from build123d import *

# Parameters (mm, degrees)
SKETCH1_R           = 1.75
SKETCH1_W           = 10
SKETCH1_H           = 5
SKETCH1_W_2         = 15
BOSS_EXTRUDE1_DEPTH = 5
SKETCH3_R           = 3.175
CUT_EXTRUDE1_DEPTH  = 2


with BuildPart() as part:
    # Sketch1 → Boss-Extrude1 (new body)
    with BuildSketch(Plane(origin=(0, 0, 0), x_dir=(1, 0, 0), z_dir=(0, 1, 0))):
        Polygon((3.647196653, 31.359118607), (3.647196653, 36.359118607), (13.647196653, 36.359118607), (13.647196653, 31.359118607), (53.647196653, 31.359118607), (53.647196653, 36.359118607), (63.647196653, 36.359118607), (63.647196653, 31.359118607), (93.647196653, 31.359118607), (93.647196653, 3.859118607), (63.647196653, 3.859118607), (63.647196653, -3.640881393), (93.647196653, -3.640881393), (93.647196653, -31.140881393), (63.647196653, -31.140881393), (63.647196653, -36.140881393), (53.647196653, -36.140881393), (53.647196653, -31.140881393), (13.647196653, -31.140881393), (13.647196653, -36.140881393), (3.647196653, -36.140881393), (3.647196653, -31.140881393), (-41.852803347, -31.140881393), (-41.852803347, 31.359118607), align=None)
        with Locations(Location((73.647196653, 22.609118607, 0), (0, 0, 270))):
            Circle(SKETCH1_R, mode=Mode.SUBTRACT)
        with Locations(Location((-1.352803347, 22.609118607, 0), (0, 0, 270))):
            Circle(SKETCH1_R, mode=Mode.SUBTRACT)
        with Locations(Location((73.647196653, -22.390881393, 0), (0, 0, 270))):
            Circle(SKETCH1_R, mode=Mode.SUBTRACT)
        with Locations(Location((-1.352803347, -22.390881393, 0), (0, 0, 270))):
            Circle(SKETCH1_R, mode=Mode.SUBTRACT)
        with Locations((83.647196653, -20.390881393)):
            Rectangle(SKETCH1_W, SKETCH1_H, mode=Mode.SUBTRACT)
        with Locations((-31.352803347, -22.390881393)):
            Rectangle(SKETCH1_W_2, SKETCH1_H, mode=Mode.SUBTRACT)
        with Locations((-31.352803347, 22.609118607)):
            Rectangle(SKETCH1_W_2, SKETCH1_H, mode=Mode.SUBTRACT)
        with Locations((83.647196653, 20.609118607)):
            Rectangle(SKETCH1_W, SKETCH1_H, mode=Mode.SUBTRACT)
    extrude(amount=BOSS_EXTRUDE1_DEPTH)

    # Sketch3 → Cut-Extrude1 (cut)
    with BuildSketch(Plane.XZ):
        with Locations(Location((-1.352803347, 22.390881393, 0), (0, 0, 270))):
            Circle(SKETCH3_R)
        with Locations(Location((73.647196653, 22.390881393, 0), (0, 0, 270))):
            Circle(SKETCH3_R)
        with Locations(Location((-1.352803347, -22.609118607, 0), (0, 0, 270))):
            Circle(SKETCH3_R)
        with Locations(Location((73.647196653, -22.609118607, 0), (0, 0, 270))):
            Circle(SKETCH3_R)
    extrude(amount=-CUT_EXTRUDE1_DEPTH, mode=Mode.SUBTRACT)


solid = part.part
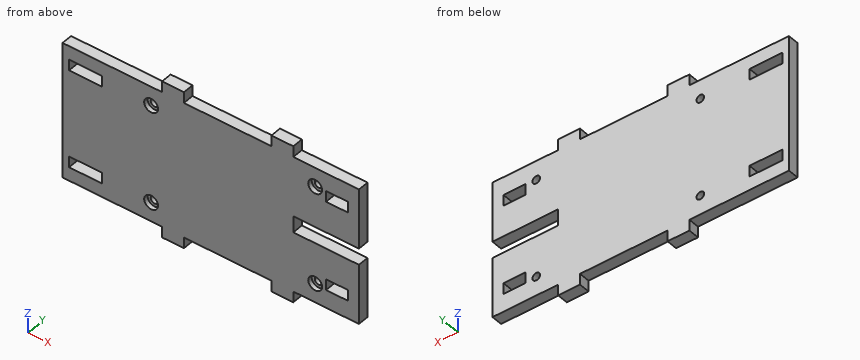
Geometry check sheet. Reference: the model listing, model coordinates, mm. Round coordinates to 2 decimals unless told otherwise and drop trailing zeros. Loops run counter-clockwise (first coordinate to the right, second up) from the corner with the lowest first, then second, coordinate; pieces in that order, holes last. Notation, with made-up numbers: (-17, 79) - (27, 79) arc R38 ccw to (27, 117) - close; hole circle Ø6 at (83.5, 89.25). An arc over 180 degrees is marked (long way). One line per question, with ' | ' between items. Start each with the question number.
1. Scan lines: line 1 (X direction, y = 4.1, z = 22.5); line 2 (Z direction, x = 84.5, y = 2.45); line 3 (Z direction, x = -25.5, y = 0.6). Record each from-to range of solid material in increasing order. Write a range as [from, to].
2. Depth check by flat-ended pin: pin 1 (2.5 mm diameter, centred on x = -34.5, y = 1.5, fed in from +Z); pin 2 (1.5 mm diameter, centred on y = 2, z = 32.5, fed in from -X). Enter the tip coordinate at first touch or a pass-through.
3. Cross-section at A-A on x = -31.5. Record the cut outline in (y, z).
4. Cross-section at D-D on x = 46. Record the cut outline in (y, z), then the cut area to 4 significant figures.
5. Cross-section at C-C on y = 3.6. State how many separate pieces and enclosed holes the cut face has, then the cut area to 3 significant figures.
6. Cross-section at B-B on x = 80. Record the cut outline in (y, z).
Taken from the geometry:
1) line 1: [-41.85, -38.85], [-23.85, -3.1], [0.39, 71.9], [75.39, 78.65], [88.65, 93.65] | line 2: [-31.36, -23.11], [-18.11, -3.86], [3.64, 17.89], [22.89, 31.14] | line 3: [-31.36, -25.11], [-20.11, 19.89], [24.89, 31.14]
2) pin 1: z = 31.14 | pin 2: x = 3.65
3) outline: (0, -31.36) - (5, -31.36) - (5, -25.11) - (0, -25.11) - close; (0, -20.11) - (5, -20.11) - (5, 19.89) - (0, 19.89) - close; (0, 24.89) - (5, 24.89) - (5, 31.14) - (0, 31.14) - close
4) outline: (0, -31.36) - (5, -31.36) - (5, 31.14) - (0, 31.14) - close | area: 312.5 mm²
5) separate pieces: 1 | enclosed holes: 8 | area: 8,160 mm²
6) outline: (0, -31.36) - (5, -31.36) - (5, -23.11) - (0, -23.11) - close; (0, -18.11) - (5, -18.11) - (5, -3.86) - (0, -3.86) - close; (0, 3.64) - (5, 3.64) - (5, 17.89) - (0, 17.89) - close; (0, 22.89) - (5, 22.89) - (5, 31.14) - (0, 31.14) - close
